Geometry: see drawing. Coordinates: mm, zero at the bounding-box minimum. A direction names the side the tool comes from. Coordinates: 2 decimals unless noted, no trailing zeros. Order: outer loops, then holes, each group sorted by start corner. A loop starts at its lowest first (then second) coordinate and runs counter-clockwise, first axis right, second up.
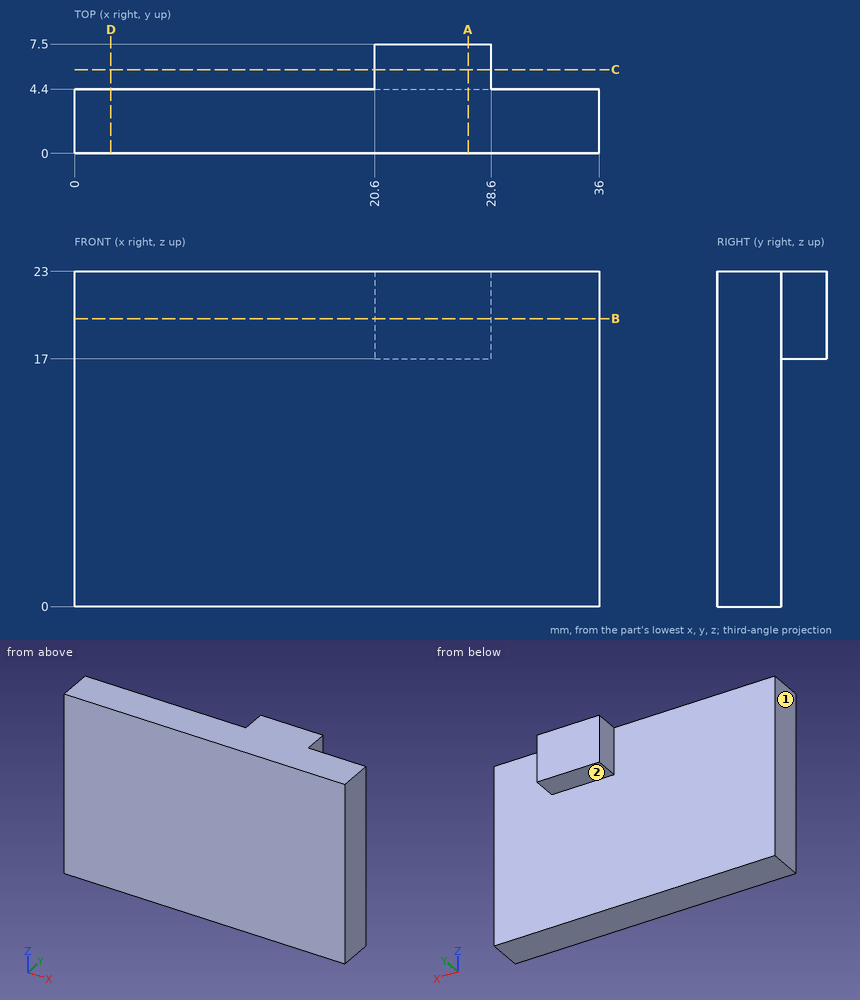
Q1. Material intervals for line 1 along X through (y, z) = (6.25, 22); line 2 along Y through (x, z) = (30.5, 3); line 3 along Z through (x, y) = (24, 4.75), sorted ascending.
Solutions:
line 1: x = 20.6 to 28.6
line 2: y = 0 to 4.4
line 3: z = 17 to 23
Q2. Section query A-A on x = 27. Output: boundary loops of the cut face in (y, z), plus the area to 3 significant figures.
Solutions:
outline: (0, 0) - (4.4, 0) - (4.4, 17) - (7.5, 17) - (7.5, 23) - (0, 23) - close
area: 120 mm2
Q3. Set-up query: the marked faces 1 and 2. Return all of +Z, -Z, +X, -X, +Y, -Y with unobstructed straight access to the full face (end or side cutting, diameter ignored); none if empty.
Solutions:
face 1: +Z, -Z, -X, +Y, -Y
face 2: -Z, +X, -X, +Y
Q4. Section query C-C on y = 5.75. Output: boundary loops of the cut face in (x, z).
Solutions:
outline: (20.6, 17) - (28.6, 17) - (28.6, 23) - (20.6, 23) - close
Q5. Section query B-B on z = 19.75. Output: boundary loops of the cut face in (x, y).
Solutions:
outline: (0, 0) - (36, 0) - (36, 4.4) - (28.6, 4.4) - (28.6, 7.5) - (20.6, 7.5) - (20.6, 4.4) - (0, 4.4) - close
Q6. Pin query (flat end, axial travel): P1, Ø6, axis at x = 19, z = 9.5, coming from the +Y side; P2, Ø2.5, axis at y = 6, z = 20, coming from the -X side; P3, Ø0.9, axis at x = 26, y = 5.5, coming from the -Z side. Return the tip coordinate at first contact, or that it passes through.
Solutions:
P1: stops at y = 4.4
P2: stops at x = 20.6
P3: stops at z = 17
Q7. Section query D-D on x = 2.5. Output: boundary loops of the cut face in (y, z).
Solutions:
outline: (0, 0) - (4.4, 0) - (4.4, 23) - (0, 23) - close
